```python
from build123d import *

# Parameters (mm, degrees)
F1_DEPTH = 38
F2_R     = 18.99999
F3_R     = 18.99999


# Not quite as in the source:
# - a fillet or chamfer is up to 0.001 mm smaller than in the source, because OpenCascade refuses the exact size


with BuildPart() as f1:
    # F0 (on Right) → F1 (new body)
    with BuildSketch(Plane.YZ):
        Polygon((-6.256232895, 31.9699999726), (-17.256232895, 31.9699999726), (-17.256232895, -18.9337489045), (39.743767105, -18.9337489045), (39.743767105, -7.9337489045), (-6.256232895, -7.9337489045), align=None)
    extrude(amount=F1_DEPTH)

    # F2 (radius 19 in the source; OpenCascade refuses exactly that, so slightly less here)
    f2_edges = [f1.edges().sort_by_distance(p)[0] for p in [
        (38, -11.756233, 31.97),
        (0, -11.756233, 31.97),
    ]]
    fillet(f2_edges, radius=F2_R)

    # F3 (radius 19 in the source; OpenCascade refuses exactly that, so slightly less here)
    f3_edges = [f1.edges().sort_by_distance(p)[0] for p in [
        (38, 39.743767, -13.433749),
        (0, 39.743767, -13.433749),
    ]]
    fillet(f3_edges, radius=F3_R)


solid = f1.part
```
Read the model definition and answer for the solid it produces. Units are mm, in the model's axes. A direction names the side the tool comes from. Round coordinates to 2 decimals unless told otherwise and drop trailing zeros. Loops run counter-clockwise (first coordinate to the right, second up) from the corner with the lowest first, then second, coordinate; pieces in that order, holes last. Notation, with made-up numbers: (25.5, -27.75) -> (46.5, -27.75) arc R27 ccw to (46.5, 3.25) -> close; hole circle Ø1 at (79.25, -39). An arc over 180 degrees is marked (long way). One line per item, written item: value.
1) For faces 1 (the face through (32.58, 34.03, -13.36)), 2 (the face through (19, 17, -7.934)), determine the directions among +Z, -Z, +X, -X, +Y, -Y from which every point of the face is accessible in a straight line to the end or side of a thin tool.
Answer list:
face 1: +Z, -Z, +X, +Y
face 2: +Z, +X, -X, +Y
2) A cutting plane is placed at B-B (x = 24). Determine the outline of the cut face in (y, z), and give its area (3 significant figures).
Answer list:
outline: (-17.26, -18.93) -> (39.07, -18.93) -> (39.07, -7.93) -> (-6.26, -7.93) -> (-6.26, 31.3) -> (-17.26, 31.3) -> close
area: 1,050 mm²
3) A cutting plane is placed at C-C (y = 1). Determine the outline of the cut face in (x, z), and give its area (3 significant figures).
Answer list:
outline: (0, -18.93) -> (38, -18.93) -> (38, -7.93) -> (0, -7.93) -> close
area: 418 mm²
4) Consider L1, parallel to Z at x = 12, y = 36; L2, parallel to Y at x = 4.5, z = -2.5; L3, parallel to X at y = 21.5, z = -14.5. Determine where each line is inside the solid, lowest interval first. Write a range as [from, to].
Answer list:
L1: z = [-18.93, -7.93]
L2: y = [-17.26, -6.26]
L3: x = [0.02, 37.98]
5) A flat-ended cylindrical pin translates along its axis: P1, Ø4, axis at x = 14, z = -5, coming from the +Y side. Find the tip coordinate at first contact, or state that the pin passes through.
Answer list:
P1: stops at y = -6.26
6) A cutting plane is placed at D-D (z = 10). Determine the outline of the cut face in (x, y).
Answer list:
outline: (0, -17.26) -> (38, -17.26) -> (38, -6.26) -> (0, -6.26) -> close
